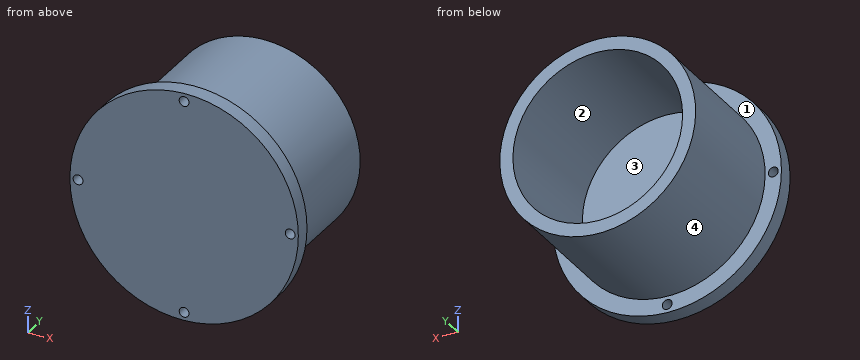
from build123d import *

# Parameters (mm, degrees)
SKETCH1_R           = 35
BOSS_EXTRUDE1_DEPTH = 5
SKETCH2_R           = 30
BOSS_EXTRUDE2_DEPTH = 40
SKETCH3_R           = 26
CUT_EXTRUDE2_DEPTH  = 60
SKETCH4_R           = 1.5
CUT_EXTRUDE3_DEPTH  = 60
BOSS_EXTRUDE3_START = -5
SKETCH5_R           = 26
BOSS_EXTRUDE3_DEPTH = 5


with BuildPart() as part:
    # Sketch1 → Boss-Extrude1 (new body)
    with BuildSketch(Plane(origin=(0, 0, 0), x_dir=(1, 0, 0), z_dir=(0, 1, 0))):
        with Locations(Location((0, 0, 0), (0, 0, 270))):
            Circle(SKETCH1_R)
    extrude(amount=BOSS_EXTRUDE1_DEPTH)

    # Sketch2 → Boss-Extrude2 (add)
    with BuildSketch(Plane(origin=(0, 5, 0), x_dir=(1, 0, 0), z_dir=(0, 1, 0))):
        with Locations(Location((0, 0, 0), (0, 0, 270))):
            Circle(SKETCH2_R)
    extrude(amount=BOSS_EXTRUDE2_DEPTH)

    # Sketch3 → Cut-Extrude2 (cut)
    with BuildSketch(Plane(origin=(0, 45, 0), x_dir=(1, 0, 0), z_dir=(0, 1, 0))):
        with Locations(Location((0, 0, 0), (0, 0, 270))):
            Circle(SKETCH3_R)
    extrude(amount=-CUT_EXTRUDE2_DEPTH, mode=Mode.SUBTRACT)

    # Sketch4 → Cut-Extrude3 (cut)
    with BuildSketch(Plane.XZ):
        with Locations(Location((0, 32.5, 0), (0, 0, 270))):
            Circle(SKETCH4_R)
        with Locations(Location((32.5, 0, 0), (0, 0, 270))):
            Circle(SKETCH4_R)
        with Locations(Location((0, -32.5, 0), (0, 0, 270))):
            Circle(SKETCH4_R)
        with Locations(Location((-32.5, 0, 0), (0, 0, 270))):
            Circle(SKETCH4_R)
    extrude(amount=-CUT_EXTRUDE3_DEPTH, mode=Mode.SUBTRACT)

    # Sketch5 → Boss-Extrude3 (add)
    with BuildSketch(Plane.XZ.offset(BOSS_EXTRUDE3_START)):
        with Locations(Location((0, 0, 0), (0, 0, 90))):
            Circle(SKETCH5_R)
    extrude(amount=BOSS_EXTRUDE3_DEPTH)


solid = part.part
Part model, mm, in its own coordinate system. Face numbers are marked on the shaded views. Coordinates: 2 decimals unless noted, no trailing zeros. Loops run counter-clockwise (first coordinate to the right, second up) from the corner with the lowest first, then second, coordinate; pieces in that order, holes last. Notation, with made-up numbers: (64, -12.75) -> (95, -12.75) arc R29 cw to (95, 10.25) -> close; hole circle Ø2 at (73, 42.25). An arc over 180 degrees is marked (long way). Use a Markdown table: item, result. Add a question column.
Item 1: Band-saw the part on C-C on y = 33. Write the cut outline in (x, z), plus the area to 3 significant figures.
Item 2: Band-saw the part on A-A on z = 0. Write the cut outline in (x, y), plus the area to 3 significant figures.
Item 3: Band-saw the part on B-B on x = 0. Write the cut outline in (y, z), plus the area to 3 significant figures.
Item 4: Band-saw the part on D-D on x = 32.5. Write the cut outline in (y, z), plus the area to 3 significant figures.
Item 5: Probe probe 1 along X at (y, z) = (2, 0); probe 2 along X at (y, z) = (42, 1); probe 3 along Y at (x, z) = (-17.5, 5). List the from-to ranges inside material, lowest first.
Item 6: Flat gauge pins, fed straight in: P1, Ø8, axis at x = -15, z = 0.5, coming from the +Y side; P2, Ø6, axis at x = 3.5, y = 22.5, coming from the -Z side; P3, Ø1, axis at y = 21, z = 8, coming from the -X side; P4, Ø3, axis at x = -23.5, z = -23, coming from the -Y side. Where does each tip first touch, or does it go through?
Item 7: Pull direction X, two halves, no side cores. Call the marked faces 1, 2, 3 and 4: +X half, -X half, draft (parallel to the pull), parting line (faces both ways), or undercut.
Geometry says:
| question | item | result |
|---|---|---|
| 1 | outline | circle Ø60 at (0, 0); hole circle Ø52 at (0, 0) |
| 1 | area | 704 mm² |
| 2 | outline | (-35, 0) -> (-34, 0) -> (-34, 5) -> (-35, 5) -> close; (-31, 0) -> (31, 0) -> (31, 5) -> (30, 5) -> (30, 45) -> (26, 45) -> (26, 5) -> (-26, 5) -> (-26, 45) -> (-30, 45) -> (-30, 5) -> (-31, 5) -> close; (34, 0) -> (35, 0) -> (35, 5) -> (34, 5) -> close |
| 2 | area | 640 mm² |
| 3 | outline | (0, -35) -> (5, -35) -> (5, -34) -> (0, -34) -> close; (0, -31) -> (5, -31) -> (5, -30) -> (45, -30) -> (45, -26) -> (5, -26) -> (5, 26) -> (45, 26) -> (45, 30) -> (5, 30) -> (5, 31) -> (0, 31) -> close; (0, 34) -> (5, 34) -> (5, 35) -> (0, 35) -> close |
| 3 | area | 640 mm² |
| 4 | outline | (0, -12.99) -> (5, -12.99) -> (5, -1.5) -> (0, -1.5) -> close; (0, 1.5) -> (5, 1.5) -> (5, 12.99) -> (0, 12.99) -> close |
| 4 | area | 115 mm² |
| 5 | probe 1 | -35 to -34, -31 to 31, 34 to 35 |
| 5 | probe 2 | -29.98 to -25.98, 25.98 to 29.98 |
| 5 | probe 3 | 0 to 5 |
| 6 | P1 | y = 5 |
| 6 | P2 | z = -30 |
| 6 | P3 | x = -29.05 |
| 6 | P4 | y = 0 |
| 7 | face 1 | draft |
| 7 | face 2 | undercut |
| 7 | face 3 | undercut |
| 7 | face 4 | parting line |
